The model under review builds one solid part; all positions refer to its coordinate system, in mm. A direction names the side the tool comes from. Give positions to 0.01 mm unless a question says otherwise; leave off trailing zeros. Order: outer loops, then holes, each group sorted by start corner. A loop starts at its lowest first (then second) coordinate and runs counter-clockwise, first axis right, second up. Notation, with made-up numbers: (19.25, -19) - (70.25, -19) arc R9 cw to (70.25, -3) - close; hole circle Ø7 at (88.25, -1). An arc over 180 degrees is marked (long way). Answer as CSV lines item,"result". Start each with the question number.
Autodesk Inventor part; units mm, degrees
ref_plane "YZ Plane" through (0, 0, 0) normal (1, 0, 0) x (0, 1, 0)
ref_plane "XZ Plane" through (0, 0, 0) normal (0, 1, 0) x (-1, 0, 0)
ref_plane "XY Plane" through (0, 0, 0) normal (0, 0, 1) x (1, 0, 0)
sketch "Sketch1" plane through (0, 0, 0) normal (0, 0, 1) x (1, 0, 0)
  line L0 (-18.76, 0) -> (18.76, 0) construction
  line L1 (0, -24.92) -> (0, 24.92) construction
  line L2 (-13.4, 17.8) -> (13.4, 17.8)
  line L3 (13.4, 17.8) -> (13.4, -17.8)
  line L4 (13.4, -17.8) -> (-13.4, -17.8)
  line L5 (-13.4, -17.8) -> (-13.4, 17.8)
  point P0 (0, 0)
  point P1 (13.4, 0)
  point P2 (0, 17.8)
  dimension "d0" = 26.8
  dimension "d1" = 35.6
extrude "Extrusion1" add sketch "Sketch1" along normal blind 1.6
sketch "Sketch3" plane through (0, 0, 1.6) normal (0, 0, 1) x (1, 0, 0)
  line L0 (5.1, 15.8) -> (11.9, 15.8)
  line L1 (11.9, 15.8) -> (11.9, 11.2)
  line L2 (11.9, 11.2) -> (5.1, 11.2)
  line L3 (5.1, 11.2) -> (5.1, 15.8)
  line L4 (13.4, 17.8) -> (-13.4, 17.8)
  line L5 (13.4, -17.8) -> (13.4, 17.8)
  point P0 (0, 0)
  dimension "d4" = 2
  dimension "d5" = 1.5
  dimension "d6" = 6.8
  dimension "d7" = 4.6
extrude "Extrusion2" add sketch "Sketch3" along normal blind 7.3
sketch "Sketch4" plane through (0, 0, 8.9) normal (0, 0, 1) x (1, 0, 0)
  circle A0 centre (10.9, 12.2) radius 0.85
  line L0 (5.1, 11.2) -> (11.9, 11.2)
  line L1 (11.9, 11.2) -> (11.9, 15.8)
  point P0 (0, 0)
  dimension "d10" = 1.7
  dimension "d11" = 1
  dimension "d12" = 1
extrude "Extrusion3" add sketch "Sketch4" along normal blind 1
sketch "Sketch5" plane through (10.9, 12.2, 9.9) normal (0, 0, 1) x (1, 0, 0)
  circle A0 centre (0, 0) radius 0.85
  line L0 (-0.25, 1.1875) -> (0.25, 1.1875)
  line L1 (0.25, 1.1875) -> (0.25, -1.2526)
  line L2 (0.25, -1.2526) -> (-0.25, -1.2526)
  line L3 (-0.25, -1.2526) -> (-0.25, 1.1875)
  point P0 (-10.9, -12.2)
  point P1 (0, -1.2526)
  dimension "d15" = 0.5
extrude "Extrusion4" cut sketch "Sketch5" against normal blind 0.5 contours L1 A0 L3 | A0 L3 L0 L1 | L1 L2 L3 A0
sketch "Sketch6" plane through (0, 0, 0) normal (0, 1, 0) x (-1, 0, 0)
  line L0 (19.9, 1.3) -> (10.4, 1.3)
  line L1 (10.4, 1.3) -> (10.4, 3.8)
  line L2 (10.4, 3.8) -> (19.9, 3.8)
  line L3 (19.9, 3.8) -> (19.9, 1.3)
  line L4 (-13.4, 1.6) -> (13.4, 1.6)
  line L5 (13.4, 0) -> (13.4, 1.6)
  point P0 (0, 0)
  dimension "d18" = 0.3
  dimension "d19" = 2.5
  dimension "d20" = 6.5
  dimension "d21" = 3
extrude "Extrusion5" add sketch "Sketch6" along normal mid plane 30
equation "\"d12\" = d11"
properties part number "P121" material "ABS Plastic"
Item 1: Take a section at D-D on z = 4.75. Write out the cut boundary in (x, y), and give its area (3 significant figures).
Item 2: Take a section at A-A on y = -5.5. Write out the cut boundary in (x, z), and give its area (3 significant figures).
Item 3: Take a section at C-C on y = 12.2. Write out the cut boundary in (x, z), and give its area (3 significant figures).
Item 4: Machinability: for faces 1 (the face through (11.685, 12.526, 9.393)), 2 (the face through (8, 15.8, 5)), 3 (the face through (9, 11.2, 5)), 4 (the face through (-17, 0, 1.3)), 5 (the face through (11.9, 14, 5)), which of the approach directions +Z, -Z, +X, -X, +Y, -Y give a long, thin tool a straight path to every point of the face, cutting with its end or side? Answer none if there is none.
Item 5: Clearance check with flat-ended pins moving along their axes: pin 1 (1 mm diameter, centred on x = -15.5, y = -12.5, fed in from -Z); pin 2 (2 mm diameter, centred on y = -10, z = 4, fed in from +X); pin 3 (7.5 mm diameter, centred on x = -15.5, y = 4.5, fed in from +Z); pin 4 (10 mm diameter, centred on x = -14, y = 14, fed in from -Z). State where each tip first meets the part, or that it passes through.
Item 6: For line 1 along X through (y, z) = (3.5, 1.75); line 2 along Y through (x, z) = (-15.5, 2.75); line 3 along X through (y, z) = (-13, 1), list the stretches that pass through material, from the lowest coordinate up.
Item 7: Take a section at B-B on x = 9. Write out the cut boundary in (y, z), and give its area (3 significant figures).
Data:
1,outline,"(5.1, 11.2) - (11.9, 11.2) - (11.9, 15.8) - (5.1, 15.8) - close"
1,area,"31.3 mm^2"
2,outline,"(-19.9, 1.3) - (-13.4, 1.3) - (-13.4, 0) - (13.4, 0) - (13.4, 1.6) - (-10.4, 1.6) - (-10.4, 3.8) - (-19.9, 3.8) - close"
2,area,"65.7 mm^2"
3,outline,"(-19.9, 1.3) - (-13.4, 1.3) - (-13.4, 0) - (13.4, 0) - (13.4, 1.6) - (11.9, 1.6) - (11.9, 8.9) - (11.75, 8.9) - (11.75, 9.9) - (11.15, 9.9) - (11.15, 9.4) - (10.65, 9.4) - (10.65, 9.9) - (10.05, 9.9) - (10.05, 8.9) - (5.1, 8.9) - (5.1, 1.6) - (-10.4, 1.6) - (-10.4, 3.8) - (-19.9, 3.8) - close"
3,area,"117 mm^2"
4,face 1,"+Z"
4,face 2,"+Z, +X, -X, +Y"
4,face 3,"+Z, +X, -Y"
4,face 4,"-Z, -X, +Y, -Y"
4,face 5,"+Z, +X, +Y, -Y"
5,pin 1,"stops at z = 1.3"
5,pin 2,"stops at x = -10.4"
5,pin 3,"stops at z = 3.8"
5,pin 4,"stops at z = 0"
6,line 1,"x = -19.9 to -10.4"
6,line 2,"y = -15 to 15"
6,line 3,"x = -13.4 to 13.4"
7,outline,"(-17.8, 0) - (17.8, 0) - (17.8, 1.6) - (15.8, 1.6) - (15.8, 8.9) - (11.2, 8.9) - (11.2, 1.6) - (-17.8, 1.6) - close"
7,area,"90.5 mm^2"
